Can you work these out from the model? Positions are in its coordinate system, mm. A direction names the side the tool comes from. Round coordinates to 2 decimals unless told otherwise and drop trailing zeros. Order: outer loops, then holes, each group sorted by start corner. A loop starts at its lowest first (then second) coordinate and runs counter-clockwise, first axis right, second up. Notation, with made-up numbers: (48.5, -24.5) - (59.5, -24.5) arc R34 ccw to (59.5, 6.5) - close; hole circle Ø4 at (64, -38). An arc over 180 degrees is marked (long way). Write item = value, one per line.
Solid Edge part; units mm, degrees
sketch "Sketch1" plane through (0, 0, 0) normal (0, 0, 1) x (1, 0, 0)
  circle A0 centre (0, 0) radius 4
extrude "Protrusion1" add sketch "Sketch1" along normal mid plane 16
chamfer "Chamfer1" distance 0.6 angle 45 2 edges at (-4, 0, -8) (-4, 0, 8)
sketch "Sketch2" plane through (0, 0, 8) normal (0, 0, 1) x (1, 0, 0)
  line L0 (-1.1547, 2) -> (1.1547, 2)
  line L1 (2.3094, 0) -> (1.1547, 2)
  line L2 (1.1547, -2) -> (2.3094, 0)
  line L3 (-1.1547, -2) -> (1.1547, -2)
  line L4 (-2.3094, 0) -> (-1.1547, -2)
  line L5 (-1.1547, 2) -> (-2.3094, 0)
extrude "Cutout1" cut sketch "Sketch2" against normal blind 8
properties part number "24104727"
(1) If we section it at A-A (z = 1.25): Write out the boundary of the cut face in (x, y).
Computed:
outline = circle Ø8 at (0, 0); hole (-2.31, 0) - (-1.15, -2) - (1.15, -2) - (2.31, 0) - (1.15, 2) - (-1.15, 2) - close
(2) Will these pins go through, and if not, where does the flat tip stop? P1, Ø3, axis at y = 0.5, z = 0, coming from the +X side; P2, Ø1.5, axis at x = -2, z = -6, coming from the -Y side; P3, Ø1.5, axis at y = -1, z = -1.5, coming from the -X side.
Computed:
P1 = 4
P2 = -3.8
P3 = -3.99
(3) On a 3-axis mill with a long thin cutter (end or side, diameter ignored), from which of +Z, -Z, +X, -X, +Y, -Y can I reach the whole of each face in a straight line? I mean faces 4 (the face through (-1.74, -0.99, 4.06)), 5 (the face through (-2, -1, 8)). Say none if no direction works.
Computed:
face_4 = +Z
face_5 = +Z, +X, -X, +Y, -Y
(4) If we section it at C-C (z = -3.75): Write out the boundary of the cut face in (x, y), plus the area to 3 significant figures.
Computed:
outline = circle Ø8 at (0, 0)
area = 50.3 mm^2
(5) If I drill on line 1 (X direction, y = 0.25, z = 1); line 2 (X direction, y = 1.5, z = 3); line 3 (Z direction, x = -0.5, y = -1), over which ranges is the centre line in solid material (lowest first)? Write a range as from..to.
Computed:
line_1 = -3.99..-2.17, 2.17..3.99
line_2 = -3.71..-1.44, 1.44..3.71
line_3 = -8..0
(6) If we section it at B-B (x = 0): Write out the boundary of the cut face in (y, z), plus the area to 3 significant figures.
Computed:
outline = (-4, -7.4) - (-3.4, -8) - (3.4, -8) - (4, -7.4) - (4, 7.4) - (3.4, 8) - (2, 8) - (2, 0) - (-2, 0) - (-2, 8) - (-3.4, 8) - (-4, 7.4) - close
area = 95.3 mm^2
(7) Thinking about a two-plate mould opening in X: for faces 1 (the face through (0, 0, -8)), 2 (the face through (1.724, -1.014, 4.056)), 3 (the face through (-0.867, -3.905, 0.104)), which applies, +X half, -X half, draft (parallel to the pull), parting line (faces both ways), or undercut?
Computed:
face_1 = draft
face_2 = undercut
face_3 = parting line
